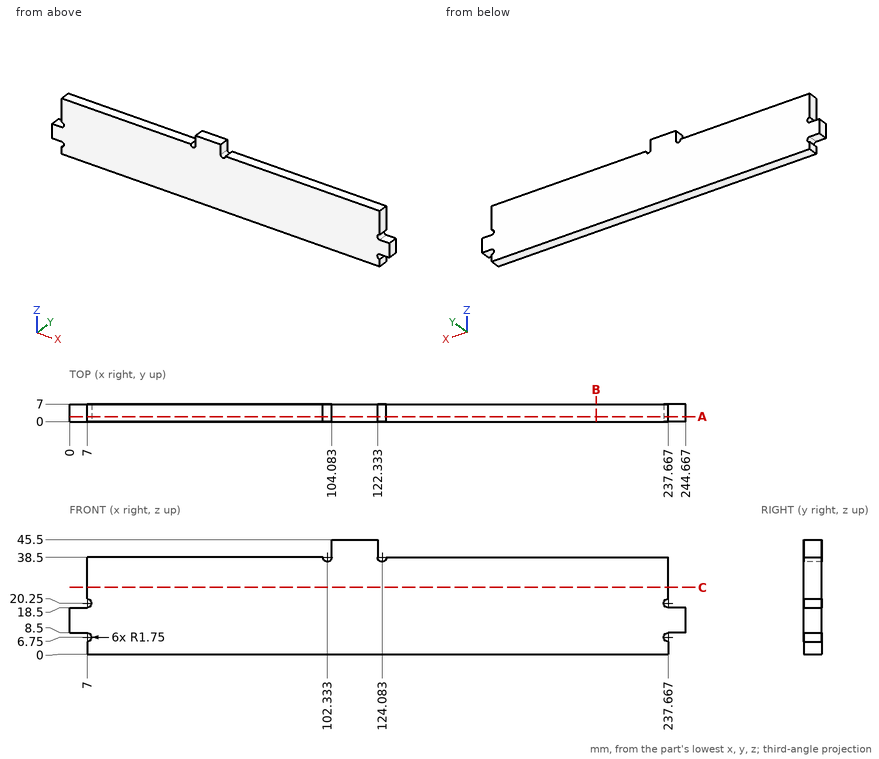
Could you check a few things on this drawing? It's one solid part, dimensions in mm from its lowest x, y, z. Give positions to 0.01 mm unless a question says otherwise; leave off trailing zeros. Loops run counter-clockwise (first coordinate to the right, second up) from the corner with the lowest first, then second, coordinate; pieces in that order, holes last. Notation, with made-up numbers: M 45.25,-36.75 L 59.25,-36.75 A13 ccw 59.25,-26.75 Z; hole C -13.5,-16.5 d6. An arc over 180 degrees is marked long. Return JSON: item names as keys, results as strings.
Item 1: Imagine slicing it at C-C on z = 26.5. List the corners of the cut face in (x, y) for me.
A:
{"outline": "M 7,0 L 237.67,0 L 237.67,7 L 7,7 Z"}
Item 2: Imagine slicing it at B-B on x = 209. List the corners of the cut face in (y, z) for me.
A:
{"outline": "M 0,0 L 7,0 L 7,38.5 L 0,38.5 Z"}
Item 3: Imagine slicing it at A-A on y = 2. List the corners of the cut face in (x, z) for me, then the cut area to 3 significant figures.
A:
{"outline": "M 0,8.5 L 7,8.5 A1.75 cw 7,5 L 7,0 L 237.67,0 L 237.67,5 A1.75 cw 237.67,8.5 L 244.67,8.5 L 244.67,18.5 L 237.67,18.5 A1.75 cw 237.67,22 L 237.67,38.5 L 125.83,38.5 A1.75 cw 122.33,38.5 L 122.33,45.5 L 104.08,45.5 L 104.08,38.5 A1.75 cw 100.58,38.5 L 7,38.5 L 7,22 A1.75 cw 7,18.5 L 0,18.5 Z", "area": "9,120 mm^2"}
Item 4: I'm going to push flat-ended pins straight in: pin 1 Ø2.5 at (y, z) = (2.5, 1.5) entering from -X; pin 2 Ø2 at (y, z) = (3.5, 41.5) entering from -X; pin 3 Ø1.5 at (y, z) = (4, 31.5) entering from +X. Where does each tip first touch, or does it pass through?
A:
{"pin 1": "stops at x = 7", "pin 2": "stops at x = 104.08", "pin 3": "stops at x = 237.67"}
Item 5: Please list where these lines run through material, in increasing order: line 1 (X direction, y = 2, z = 3.5); line 2 (X direction, y = 0.5, z = 40.5); line 3 (Z direction, x = 135, y = 1.25).
A:
{"line 1": "x = 7 to 237.67", "line 2": "x = 104.08 to 122.33", "line 3": "z = 0 to 38.5"}
